Source: three-view drawing plus pictorial views. Frame: mm from the lowest corner of the part. A direction names the side the tool comes from. Give positions to 0.01 mm unless a question says otherwise; leave off trailing zeros. Loops run counter-clockwise (first coordinate to the right, second up) from the corner with the lowest first, then second, coordinate; pieces in that order, holes last.
1. Material intervals for line 1 along X through (y, z) = (12.75, 6); line 2 along Z through (x, y) = (12.85, 5); line 3 along Y through (x, z) = (4, 1), sorted ascending.
2. Section A-A, the plane x = 6.5. Output: boundary loops of the cut face in (y, z), then the cut area to 3 significant figures.
3. First-contact query: P1, Ø3, axis at x = 6, z = 3.5, coming from the -Y side. Flat tip, straight axial feed; report the tip coordinate or a pass-through.
4. Section B-B, the plane y = 15. Output: boundary loops of the cut face in (x, z), then the cut area to 3 significant figures.
5. Draft query along X for the marked faces 1, 2, 3 and 4. Return one class per face: +X half, -X half, draft (parallel to the pull), parting line (faces both ways), or undercut.
6. Access query for the marked faces 5 and 6. Directions: +Z, -Z, +X, -X, +Y, -Y. A direction counts if a zero-diameter tool reaches every point of the face in a straight line with its end or side. Return the directions, or none.
7. Section D-D, the plane z = 6.5. State how many separate pieces and enclosed holes the cut face has, then the cut area to 3 significant figures.
8. Section C-C, the plane y = 9.5. Output: boundary loops of the cut face in (x, z), then the cut area to 3 significant figures.
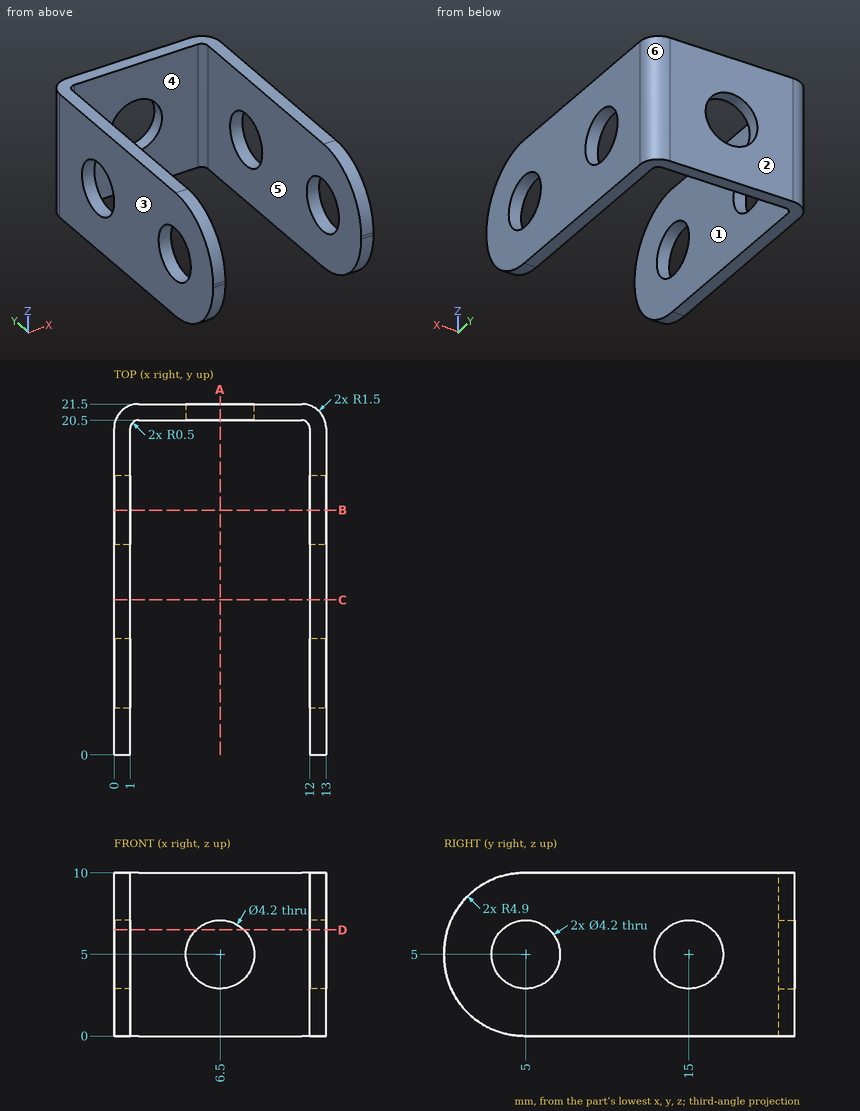
Answers below:
1. line 1: x = 0 to 1, 12 to 13
1. line 2: z = 0 to 2.9, 7.1 to 10
1. line 3: y = 20.5 to 21.5
2. outline: (20.5, 0) - (21.5, 0) - (21.5, 2.9) - (20.5, 2.9) - close; (20.5, 7.1) - (21.5, 7.1) - (21.5, 10) - (20.5, 10) - close
2. area: 5.80 mm2
3. P1: stops at y = 20.5
4. outline: (0, 0) - (1, 0) - (1, 2.9) - (0, 2.9) - close; (0, 7.1) - (1, 7.1) - (1, 10) - (0, 10) - close; (12, 0) - (13, 0) - (13, 2.9) - (12, 2.9) - close; (12, 7.1) - (13, 7.1) - (13, 10) - (12, 10) - close
4. area: 11.6 mm2
5. face 1: undercut
5. face 2: draft
5. face 3: -X half
5. face 4: undercut
6. face 5: +Z, -Z, -Y
6. face 6: +Z, -Z, +X, +Y
7. separate pieces: 6
7. enclosed holes: 0
7. area: 38.0 mm2
8. outline: (0, 0) - (1, 0) - (1, 10) - (0, 10) - close; (12, 0) - (13, 0) - (13, 10) - (12, 10) - close
8. area: 20.0 mm2
